from build123d import *

# Parameters (mm, degrees)
F0_R     = 85
F2_R     = 0.5
F4_R     = 105.9677495378
F5_DEPTH = 1


# Not quite as in the source:
# - a fillet or chamfer that OpenCascade refuses, or shapes differently, is made with other operations: its cross-section is extruded or revolved along the edge and cut away or added


with BuildPart() as f3:
    # F0 (on Top) → F3 section 0
    with BuildSketch(Plane.XY):
        Circle(F0_R)
    # F2 (on offset) → F3 section 1
    with BuildSketch(Plane.XY.offset(1100)):
        Circle(F2_R)
    loft()

    # F4 (on Top) → F5 (join)
    with BuildSketch(Plane.XY):
        Circle(F4_R)
    extrude(amount=F5_DEPTH)

    # F6: fillet of radius 50 on 1 edges, made by hand


with BuildPart() as f6_tool2:
    # F6_s3 → F6_t4 (revolve)
    with BuildSketch(Plane.XZ):
        with BuildLine():
            ThreePointArc((105.9675430277, 0.9996574309), (89.2196248611, 17.5811287524), (81.9274601503, 39.9923377321))
            Line((81.9274601503, 39.9923377321), (76.9419980029, 39.6093635944))
            ThreePointArc((76.9419980029, 39.6093635944), (78.4400582493, 20.1132100469), (79.9377196708, 0.6170258623))
            Line((79.9377196708, 0.6170258623), (84.9231818182, -4.0001501991))
            ThreePointArc((84.9231818182, -4.0001501991), (95.4453624229, -4.0001501991), (103.386089168, -3.2825847369))
            Line((103.386089168, -3.2825847369), (105.9675430277, 0.9996574309))
        make_face()
    revolve(axis=Axis((0, 0, 1), (0, 0, 1)))

    split(bisect_by=Plane.XY, keep=Keep.TOP)


with BuildPart() as f3_1:
    add(f3.part)

    # F6_t1: union F6_tool2
    add(f6_tool2.part)


solid = f3_1.part
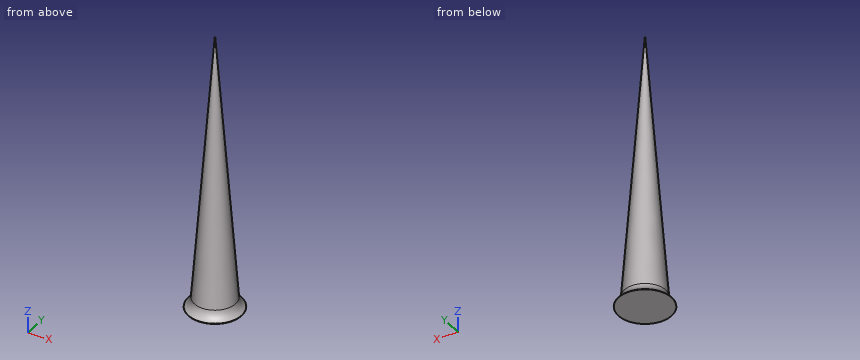
The listing builds one solid part. Answer for the finished solid, in the listing's coordinates (mm). Round coordinates to 2 decimals unless told otherwise and drop trailing zeros. Write each loop counter-clockwise with the first axis right and the second up, starting at its lowest first coordinate (ties: lowest second). Pieces come first, ordered by that corner, then holes. Notation, with made-up numbers: M 87,62 L 133,62 A15 cw 133,81 Z; hole C 84.25,-34.75 d1. An arc over 180 degrees is marked long. Write each question's results on one line, items separated by ' | '. Start each with the question number.
(1) The part is cut by section B-B, the plane z = 712. Write down the section's boundary in (x, y), and give its area (3 significant figures).
(2) The part is cut by section A-A, the plane z = 349. Write down the section's boundary in (x, y), and give its area (3 significant figures).
(3) Find the intervals of material crossed by line 1 (X direction, y = -7, z = 955); line 2 (X direction, y = 1, z = 608.5); line 3 (Z direction, x = -84.5, y = 15), in increasing order.
(4) This flat-tipped pin is pushed along its axis until it touches: P1, Ø10, axis at y = -34, z = 614.5, coming from the +X side. Where does it stop, or does it pass through?
Worked answers:
1) outline: C 0,0 d60.61 | area: 2,890 mm²
2) outline: C 0,0 d116.38 | area: 10,600 mm²
3) line 1: x = -9.3 to 9.3 | line 2: x = -38.24 to 38.24 | line 3: z = 0 to 24.13
4) P1: stops at x = 24.27
